Check sheet for the modelled part. Datum: model origin and axes. Units: mm. A direction names the side the tool comes from. Round coordinates to 2 decimals unless told otherwise and drop trailing zeros. Loops run counter-clockwise (first coordinate to the right, second up) from the corner with the lowest first, then second, coordinate; pieces in that order, holes last. Notation, with made-up numbers: (-34, 89) -> (-30, 89) arc R19 cw to (-30, 122) -> close; hole circle Ø5 at (-2.75, 18.5). An arc over 180 degrees is marked (long way). One line per item, written item: value. Start each with the question number.
1. Set-up check for faces 4 (the face through (4, 5, -6)), 5 (the face through (1, 4, -7.333)), 6 (the face through (11, 4, -6)): record each of +Z, -Z, +X, -X, +Y, -Y from which the full face is reachable in a straight line by a thin tool's end or side.
2. Cross-section at C-C on z = -2.25. Record the cut outline in (x, y), then the cut area to 3 significant figures.
3. Cross-section at B-B on x = 4.75. Record the cut outline in (y, z).
4. Cross-section at A-A on z = -7. Record the cut outline in (x, y).
5. Go/stop test with a flat-tipped pin: pin 1 (1 mm diameter, centred on x = 1, y = 3.5, fed in from +Z). Record where the tip stops, or that it passes through.
6. Cross-section at D-D on x = 2.75. Record the cut outline in (y, z).
7. Release check for a two-part mould opening along X. For faces 1 (the face through (13, 4, -2.667)), 2 (the face through (12, 4, -9)), 3 (the face through (0, 2, -5)) record: +X half, -X half, draft (parallel to the pull), parting line (faces both ways), or undercut.
8. Material ranges on L1, parallel to Z at x = 6.75, y = 3.95; L2, parallel to X at y = 4.35, z = -7; L3, parallel to Y at x = 5.5, z = -9.25, recorded low to high.
from build123d import *

# Parameters (mm, degrees)
SKETCH1_W           = 14
SKETCH1_H           = 10
BOSS_EXTRUDE1_DEPTH = 3
SKETCH2_W           = 2
SKETCH2_H           = 2
BOSS_EXTRUDE2_DEPTH = 2


with BuildPart() as part:
    # Sketch1 → Boss-Extrude1 (new body)
    with BuildSketch(Plane(origin=(0, 0, 0), x_dir=(1, 0, 0), z_dir=(0, 1, 0))):
        with Locations((7, 5)):
            Rectangle(SKETCH1_W, SKETCH1_H)
    extrude(amount=BOSS_EXTRUDE1_DEPTH)

    # Sketch2 → Boss-Extrude2 (add)
    with BuildSketch(Plane(origin=(0, 3, 0), x_dir=(1, 0, 0), z_dir=(0, 1, 0))):
        with Locations((4, 1)):
            Rectangle(SKETCH2_W, SKETCH2_H)
        with Locations((1, 1)):
            Rectangle(SKETCH2_W, SKETCH2_H)
        with Locations((7, 1)):
            Rectangle(SKETCH2_W, SKETCH2_H)
        with Locations((10, 1)):
            Rectangle(SKETCH2_W, SKETCH2_H)
        with Locations((4, 3.666666667)):
            Rectangle(SKETCH2_W, SKETCH2_H)
        with Locations((7, 3.666666667)):
            Rectangle(SKETCH2_W, SKETCH2_H)
        with Locations((10, 3.666666667)):
            Rectangle(SKETCH2_W, SKETCH2_H)
        with Locations((4, 6.333333333)):
            Rectangle(SKETCH2_W, SKETCH2_H)
        with Locations((7, 6.333333333)):
            Rectangle(SKETCH2_W, SKETCH2_H)
        with Locations((10, 6.333333333)):
            Rectangle(SKETCH2_W, SKETCH2_H)
        with Locations((4, 9)):
            Rectangle(SKETCH2_W, SKETCH2_H)
        with Locations((7, 9)):
            Rectangle(SKETCH2_W, SKETCH2_H)
        with Locations((10, 9)):
            Rectangle(SKETCH2_W, SKETCH2_H)
        with Locations((1, 3.666666667)):
            Rectangle(SKETCH2_W, SKETCH2_H)
        with Locations((1, 6.333333333)):
            Rectangle(SKETCH2_W, SKETCH2_H)
        with Locations((1, 9)):
            Rectangle(SKETCH2_W, SKETCH2_H)
        with Locations((13, 1)):
            Rectangle(SKETCH2_W, SKETCH2_H)
        with Locations((13, 3.666666667)):
            Rectangle(SKETCH2_W, SKETCH2_H)
        with Locations((13, 6.333333333)):
            Rectangle(SKETCH2_W, SKETCH2_H)
        with Locations((13, 9)):
            Rectangle(SKETCH2_W, SKETCH2_H)
    extrude(amount=BOSS_EXTRUDE2_DEPTH)


solid = part.part
Taken from the geometry:
1. face 4: +Z, -Z, +X, -X, +Y
1. face 5: +X, -X, +Y
1. face 6: +Z, -Z, +Y
2. outline: (0, 0) -> (14, 0) -> (14, 3) -> (0, 3) -> close
2. area: 42.0 mm2
3. outline: (0, -10) -> (5, -10) -> (5, -8) -> (3, -8) -> (3, -7.33) -> (5, -7.33) -> (5, -5.33) -> (3, -5.33) -> (3, -4.67) -> (5, -4.67) -> (5, -2.67) -> (3, -2.67) -> (3, -2) -> (5, -2) -> (5, 0) -> (0, 0) -> close
4. outline: (0, 0) -> (14, 0) -> (14, 5) -> (12, 5) -> (12, 3) -> (11, 3) -> (11, 5) -> (9, 5) -> (9, 3) -> (8, 3) -> (8, 5) -> (6, 5) -> (6, 3) -> (5, 3) -> (5, 5) -> (3, 5) -> (3, 3) -> (2, 3) -> (2, 5) -> (0, 5) -> close
5. pin 1: stops at z = 0
6. outline: (0, -10) -> (3, -10) -> (3, 0) -> (0, 0) -> close
7. face 1: draft
7. face 2: undercut
7. face 3: -X half
8. L1: z = -10 to -8, -7.33 to -5.33, -4.67 to -2.67, -2 to 0
8. L2: x = 0 to 2, 3 to 5, 6 to 8, 9 to 11, 12 to 14
8. L3: y = 0 to 3
